Work out the finished part from the listing and answer in its coordinate system (mm). Face numbers are marked on the shaded views. A direction names the side the tool comes from. Round coordinates to 2 decimals unless told otherwise and drop trailing zeros. Write each loop counter-clockwise with the first axis right and the second up, starting at its lowest first coordinate (ties: lowest second). Pieces come first, ordered by that corner, then holes. Notation, with made-up numbers: M 83.25,11 L 139.25,11 A20 cw 139.25,23 Z; hole C 12,29 d6. An arc over 180 degrees is marked long. Answer in a Markdown table with one row per item.
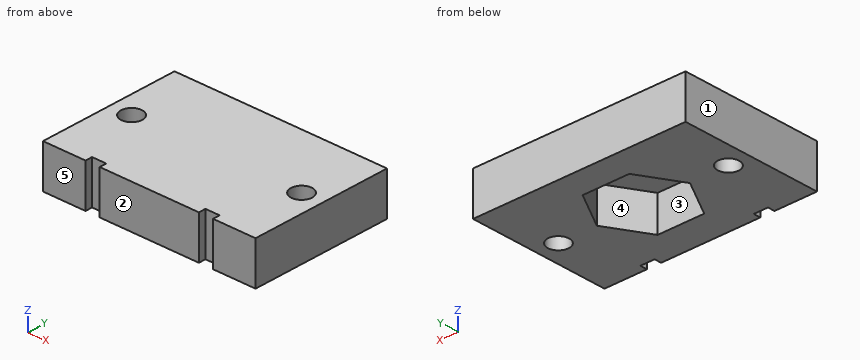
```python
from build123d import *

# Parameters (mm, degrees)
CROQUIS1_W                 = 15
CROQUIS1_H                 = 10
SALIENTE_EXTRUIR1_DEPTH    = 1.5
CORTAR_EXTRUIR2_DEPTH      = 1
CORTAR_EXTRUIR2_DEPTH_BACK = 13.589678312
CROQUIS4_W                 = 1
CROQUIS4_H                 = 3
CORTAR_EXTRUIR3_DEPTH      = 0.5
CROQUIS6_R                 = 0.75
CORTAR_EXTRUIR6_DEPTH      = 13.854960132


with BuildPart() as part:
    # Croquis1 → Saliente-Extruir1 (new, symmetric)
    with BuildSketch(Plane.XY):
        with Locations((0, 5)):
            Rectangle(CROQUIS1_W, CROQUIS1_H)
    extrude(amount=SALIENTE_EXTRUIR1_DEPTH, both=True)

    # Croquis3 → Cortar-Extruir2 (cut, two sides: drawn at the far end of the back side and taken through both)
    with BuildSketch(Plane.XY.offset(-CORTAR_EXTRUIR2_DEPTH_BACK)):
        Polygon((3.290896534, 5.12), (1.645448267, 7.97), (-1.645448267, 7.97), (-3.290896534, 5.12), (-1.645448267, 2.27), (1.645448267, 2.27), align=None)
    extrude(amount=CORTAR_EXTRUIR2_DEPTH + CORTAR_EXTRUIR2_DEPTH_BACK, mode=Mode.SUBTRACT)

    # Croquis4 → Cortar-Extruir3 (cut)
    with BuildSketch(Plane.XZ):
        with Locations((-4, 0)):
            Rectangle(CROQUIS4_W, CROQUIS4_H)
        with Locations((4, 0)):
            Rectangle(CROQUIS4_W, CROQUIS4_H)
    extrude(amount=-CORTAR_EXTRUIR3_DEPTH, mode=Mode.SUBTRACT)

    # Croquis6 → Cortar-Extruir6 (cut, through all)
    with BuildSketch(Plane(origin=(0, 0, -1.5), x_dir=(-1, 0, 0), z_dir=(0, 0, -1))):
        with Locations((-6, 5.12)):
            Circle(CROQUIS6_R)
        with Locations((6, 5.12)):
            Circle(CROQUIS6_R)
    extrude(amount=-CORTAR_EXTRUIR6_DEPTH, mode=Mode.SUBTRACT)


solid = part.part
```
1. A tool of negligible diameter and unlimited length cuts with its end or side. For the marked faces 4 and 5, from which of +Z, -Z, +X, -X, +Y, -Y can it reach the whole face along a straight path? Write none if from no direction.
Calculated:
| item | result |
|---|---|
| face 4 | -Z |
| face 5 | +Z, -Z, +X, -X, -Y |
2. The part is cut by section B-B (x = 6). Determine the outline of the cut face in (y, z), plus the area to 3 significant figures.
Calculated:
| item | result |
|---|---|
| outline | M 0,-1.5 L 4.37,-1.5 L 4.37,1.5 L 0,1.5 Z; M 5.87,-1.5 L 10,-1.5 L 10,1.5 L 5.87,1.5 Z |
| area | 25.5 mm² |
3. The part is cut by section A-A (z = -0.8). Determine the outline of the cut face in (x, y).
Calculated:
| item | result |
|---|---|
| outline | M -7.5,0 L -4.5,0 L -4.5,0.5 L -3.5,0.5 L -3.5,0 L 3.5,0 L 3.5,0.5 L 4.5,0.5 L 4.5,0 L 7.5,0 L 7.5,10 L -7.5,10 Z; hole C -6,5.12 d1.5; hole M -3.29,5.12 L -1.65,2.27 L 1.65,2.27 L 3.29,5.12 L 1.65,7.97 L -1.65,7.97 Z; hole C 6,5.12 d1.5 |
4. Determine the mould class of the marked faces 1, 2 and 3 for opening direction X: released by +X, released by -X, zero draft, split by the parting line, or undercut.
Calculated:
| item | result |
|---|---|
| face 1 | released by -X |
| face 2 | zero draft |
| face 3 | undercut |
5. The part is cut by section C-C (y = 3.5). Determine the outline of the cut face in (x, z), plus the area to 3 significant figures.
Calculated:
| item | result |
|---|---|
| outline | M -7.5,-1.5 L -2.36,-1.5 L -2.36,1 L 2.36,1 L 2.36,-1.5 L 7.5,-1.5 L 7.5,1.5 L -7.5,1.5 Z |
| area | 33.2 mm² |
6. Consider line 1 along Y through (x, z) = (0.5, -1.1); line 2 along Y through (x, z) = (-6, 0.1); line 3 along X through (y, z) = (4.75, -0.8). Determine where each line is inside the solid, lowest interval first. Write a range as from..to.
Calculated:
| item | result |
|---|---|
| line 1 | y = 0..2.27, 7.97..10 |
| line 2 | y = 0..4.37, 5.87..10 |
| line 3 | x = -7.5..-6.65, -5.35..-3.08, 3.08..5.35, 6.65..7.5 |
7. The part is cut by section D-D (x = 4). Determine the outline of the cut face in (y, z).
Calculated:
| item | result |
|---|---|
| outline | M 0.5,-1.5 L 10,-1.5 L 10,1.5 L 0.5,1.5 Z |
